Job drawing, mm, ordinate dimensions from the low corner. One solid piece. A direction names the side the tool comes from. Coordinates: 2 decimals unless noted, no trailing zeros. Order: outer loops, then holes, each group sorted by start corner. A loop starts at its lowest first (then second) coordinate and runs counter-clockwise, first axis right, second up. Notation, with made-up numbers: (23, 47) - (35, 47) arc R22 cw to (35, 86) - close; hole circle Ø6 at (78, -1). An arc over 180 degrees is marked (long way). Use a Markdown table: item, result. Add a question column.
1) Saw through at B-B on x = 23.5. List the corners of the cut face in (y, z) (3 decimals), then the cut area to 3 significant figures.
2) Wall check: L1, parallel to X at y = 24, z = 16.75. Give the ranges that are in metal, low to high. Write a range as [from, to].
3) Drop flat-ended pins along their axis: P1, Ø1, axis at y = 7, z = 18, coming from the +X side; P2, Ø8, axis at x = 13.5, y = 18, coming from the -Z side (3 decimals); P3, Ø12, axis at x = 80, y = 14, coming from the -Z side; P4, Ø10, axis at x = 107.5, y = 13, coming from the +Z side (3 decimals). Give the stop position or say it passes through.
4) Saw through at A-A on y = 11.25. List the corners of the cut face in (x, z) (3 decimals), then the cut area to 3 significant figures.
5) Tool access for the marked faces 1, 2, 3, 4 and 5: list every direction of +Z, -Z, +X, -X, +Y, -Y with a clear straight run to the whole face (end or side of a thin tool).
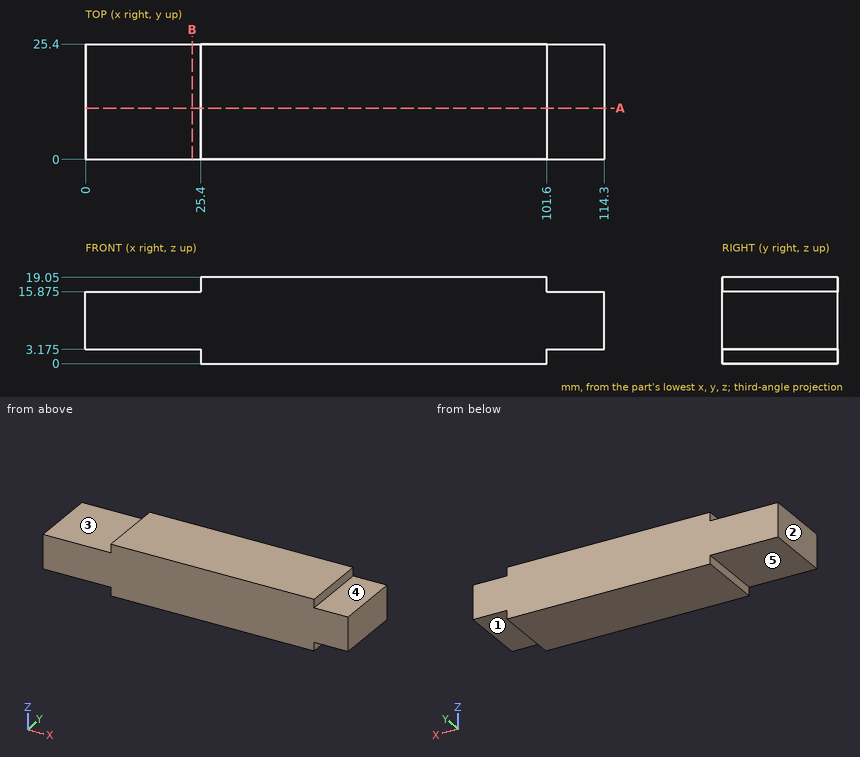
Results are:
| question | item | result |
|---|---|---|
| 1 | outline | (0, 3.175) - (25.4, 3.175) - (25.4, 15.875) - (0, 15.875) - close |
| 1 | area | 323 mm2 |
| 2 | L1 | [25.4, 101.6] |
| 3 | P1 | x = 101.6 |
| 3 | P2 | z = 3.175 |
| 3 | P3 | z = 0 |
| 3 | P4 | z = 15.875 |
| 4 | outline | (0, 3.175) - (25.4, 3.175) - (25.4, 0) - (101.6, 0) - (101.6, 3.175) - (114.3, 3.175) - (114.3, 15.875) - (101.6, 15.875) - (101.6, 19.05) - (25.4, 19.05) - (25.4, 15.875) - (0, 15.875) - close |
| 4 | area | 1,940 mm2 |
| 5 | face 1 | -Z, +X, +Y, -Y |
| 5 | face 2 | +Z, -Z, -X, +Y, -Y |
| 5 | face 3 | +Z, -X, +Y, -Y |
| 5 | face 4 | +Z, +X, +Y, -Y |
| 5 | face 5 | -Z, -X, +Y, -Y |
